Input: part model. Units: mm. Frame: model coordinates. A direction names the side the tool comes from. Round coordinates to 2 decimals unless told otherwise and drop trailing zeros. Loops run counter-clockwise (first coordinate to the right, second up) from the corner with the lowest first, then second, coordinate; pieces in that order, holes last. Notation, with made-up numbers: (72.5, 28.5) -> (96.5, 28.5) arc R29 cw to (96.5, 65.5) -> close; hole circle Ø4 at (52, 89). An arc over 180 degrees is marked (long way). Answer as a JSON object with one key per item and string values. Group by question number.
Item 1: Material intervals for line 1 (Y direction, x = -4, z = 1); line 2 (Z direction, x = 5.5, y = -8), sorted ascending. Write a range as [from, to].
Item 2: Set-up query: faces 1 (the flat face through (0, -6, 3.25)), 2 (the flat face through (-8, -2, 4)). Return all of +Z, -Z, +X, -X, +Y, -Y with unobstructed straight access to the full face (end or side cutting, diameter ignored); none if empty.
Item 3: Section query A-A on x = 1.5. Return loops of the section in (y, z), and give its area (4 significant figures).
Item 4: Section query B-B on z = 2.75. Return loops of the section in (x, y).
Item 5: Section query C-C on y = -7.5. Return loops of the section in (x, z), and give its area (3 significant figures).
Item 6: Pin query (flat end, axial travel): pin 1 (1 mm diameter, centred on x = 2, z = -1.5, fed in from -Y); pin 2 (6 mm diameter, centred on x = -2.5, y = -5.5, fed in from -Z). Return the tip coordinate at first contact, or that it passes through.
from build123d import *

# Parameters (mm, degrees)
SKETCH1_W           = 16
SKETCH1_H           = 9.5
BOSS_EXTRUDE1_DEPTH = 3.2
SKETCH2_W           = 16
SKETCH2_H           = 12.5
BOSS_EXTRUDE2_DEPTH = 1.5


with BuildPart() as part:
    # Sketch1 → Boss-Extrude1 (new body)
    with BuildSketch(Plane(origin=(0, 0, 0), x_dir=(1, 0, 0), z_dir=(0, 1, 0))):
        Rectangle(SKETCH1_W, SKETCH1_H)
    extrude(amount=BOSS_EXTRUDE1_DEPTH)

    # Sketch2 → Boss-Extrude2 (add)
    with BuildSketch(Plane.XY.offset(4.75)):
        with Locations((0, -6.25)):
            Rectangle(SKETCH2_W, SKETCH2_H)
    extrude(amount=-BOSS_EXTRUDE2_DEPTH)


solid = part.part
Solved:
{
 "1": {"line 1": "[0, 3.2]", "line 2": "[3.25, 4.75]"},
 "2": {"face 1": "-Z, +X, -X, -Y", "face 2": "+Z, -Z, -X, +Y, -Y"},
 "3": {"outline": "(-12.5, 3.25) -> (0, 3.25) -> (0, -4.75) -> (3.2, -4.75) -> (3.2, 4.75) -> (-12.5, 4.75) -> close", "area": "49.15 mm²"},
 "4": {"outline": "(-8, 0) -> (8, 0) -> (8, 3.2) -> (-8, 3.2) -> close"},
 "5": {"outline": "(-8, 3.25) -> (8, 3.25) -> (8, 4.75) -> (-8, 4.75) -> close", "area": "24.0 mm²"},
 "6": {"pin 1": "y = 0", "pin 2": "z = 3.25"}
}
